The listing builds one solid part. Answer for the finished solid, in the listing's coordinates (mm). Face numbers are marked on the shaded views. A direction names the side the tool comes from. Coordinates: 2 decimals unless noted, no trailing zeros. Loops run counter-clockwise (first coordinate to the right, second up) from the corner with the lowest first, then second, coordinate; pieces in that order, holes last. Notation, with made-up numbers: (1.5, 11.25) - (60.5, 11.25) arc R10 cw to (60.5, 22.25) - close; hole circle Ø9 at (23.5, -15). An arc over 180 degrees is marked (long way). Return JSON: item names as keys, results as strings. Group by question number.
1. Section C-C (x = 9.25) is taken. Write down the section's boundary in (y, z).
2. Find the intervals of material crossed by line 1 along X through (y, z) = (0, -2.25); line 2 along Y through (x, z) = (-3, -0.75); line 3 along Y through (x, z) = (-2.75, -4.5), in increasing order.
3. Section B-B (z = 0) is taken. Write down the section's boundary in (x, y).
4. Which of the six approach directions +Z, -Z, +X, -X, +Y, -Y give full straight-line access (tool end or side, diameter ignored) to the marked faces 4, 5 and 6?
5. Section A-A (y = 0) is taken. Write down the section's boundary in (x, z).
6. The mould has two halves that part along Y. Classify the marked faces 1, 2 and 3: pulls with the +Y half, pulls with the -Y half, needs draft (parallel to the pull), parting line crosses it, or undercut.
7. Each of these flat-tipped pins is pushed along its axis until it touches: P1, Ø8, axis at y = 3.5, z = 2, coming from the +X side; P2, Ø1, axis at x = 4, y = 0, coming from the +Z side; P3, Ø2, axis at x = 0.5, y = -3, coming from the +Z side; P4, Ø2, axis at x = 7.5, y = -4.5, coming from the +Z side. Where does it stop, or does it pass through?
8. Section D-D (x = -2.5) is taken. Write down the section's boundary in (y, z).
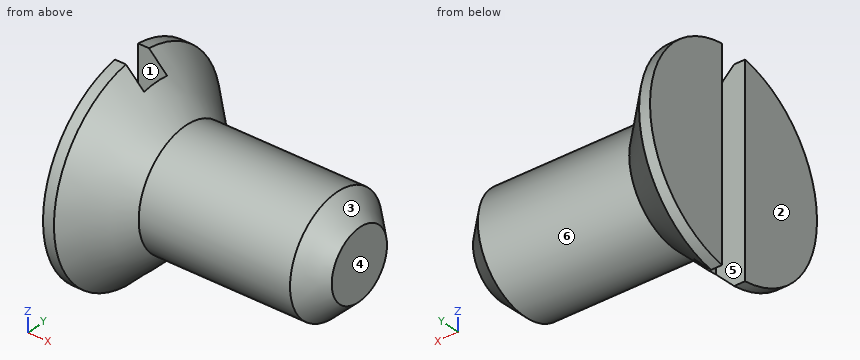
Autodesk Inventor part; units mm, degrees
ref_plane "YZ Plane" through (0, 0, 0) normal (1, 0, 0) x (0, 1, 0)
ref_plane "XZ Plane" through (0, 0, 0) normal (0, 1, 0) x (-1, 0, 0)
ref_plane "XY Plane" through (0, 0, 0) normal (0, 0, 1) x (1, 0, 0)
sketch "Эскиз1" plane through (0, 0, 0) normal (1, 0, 0) x (0, 1, 0)
  circle A0 centre (0, 0) radius 4
  dimension "d0" = 8
extrude "Выдавливание1" add sketch "Эскиз1" along normal blind 12
chamfer "Фаска1" distance 1.6 angle 45 1 edges at (12, -4, 0)
thread "Резьба1"
sketch "Эскиз2" plane through (0, 0, 0) normal (0, 0, 1) x (1, 0, 0)
  line L0 (0, 4) -> (0, -4)
  line L1 (0, 0) -> (0, 4)
  line L2 (0, 4) -> (-4, 8)
  line L3 (0, 4) -> (5.6569, 4) construction
  line L4 (-4, 8) -> (-4, 4)
  line L5 (-4, 0) -> (0, 0)
  line L6 (0, 4) -> (0, 0)
  line L7 (-4, 0) -> (-4, 4)
  dimension "d8" = 4
  dimension "d9" = 135
revolve "Вращение1" add sketch "Эскиз2" angle 360 about axis through (-4, 0, 0) along (1, 0, 0)
sketch "Эскиз3" plane through (-4, 0, 0) normal (-1, 0, 0) x (0, 0, 1)
  circle A0 centre (0, 0) radius 7.25
  dimension "d11" = 14.5
extrude "Выдавливание2" cut sketch "Эскиз3" against normal blind 25.25 keep common part
sketch "Эскиз4" plane through (0, 0, 0) normal (0, 0, 1) x (1, 0, 0)
  line L0 (-6, 1) -> (-2, 1)
  line L1 (-2, 1) -> (-2, -1)
  line L2 (-2, -1) -> (-6, -1)
  line L3 (-6, -1) -> (-6, 1)
  line L4 (-4, -7.25) -> (-4, 7.25)
  line L5 (-6, 1) -> (-2, -1) construction
  line L6 (-2, 1) -> (-6, -1) construction
  point P0 (0, 0)
  point P1 (-4, 0)
  dimension "d14" = 4
  dimension "d15" = 2
extrude "Выдавливание3" cut sketch "Эскиз4" along normal mid plane 25.25
properties part number "винт"
The answers:
{
 "1": {"outline": "circle Ø8 at (0, 0)"},
 "2": {"line 1": "x = -2 to 12", "line 2": "y = -6.96 to -1, 1 to 6.96", "line 3": "y = -5.03 to -1, 1 to 5.03"},
 "3": {"outline": "(-4, -7.25) - (-3.25, -7.25) - (0, -4) - (10.4, -4) - (12, -2.4) - (12, 2.4) - (10.4, 4) - (0, 4) - (-3.25, 7.25) - (-4, 7.25) - (-4, 1) - (-2, 1) - (-2, -1) - (-4, -1) - close"},
 "4": {"face 4": "+Z, -Z, +X, +Y, -Y", "face 5": "+Z, -Z, -X", "face 6": "+X"},
 "5": {"outline": "(-2, -6) - (0, -4) - (10.4, -4) - (12, -2.4) - (12, 2.4) - (10.4, 4) - (0, 4) - (-2, 6) - close"},
 "6": {"face 1": "undercut", "face 2": "needs draft", "face 3": "parting line crosses it"},
 "7": {"P1": "stops at x = 12", "P2": "stops at z = 4", "P3": "stops at z = 3.58", "P4": "stops at z = 1.94"},
 "8": {"outline": "(-1, -6.42) - (-1, 6.42) arc R6.5 ccw to start; (1, -6.42) arc R6.5 ccw to (1, 6.42) - close"}
}
